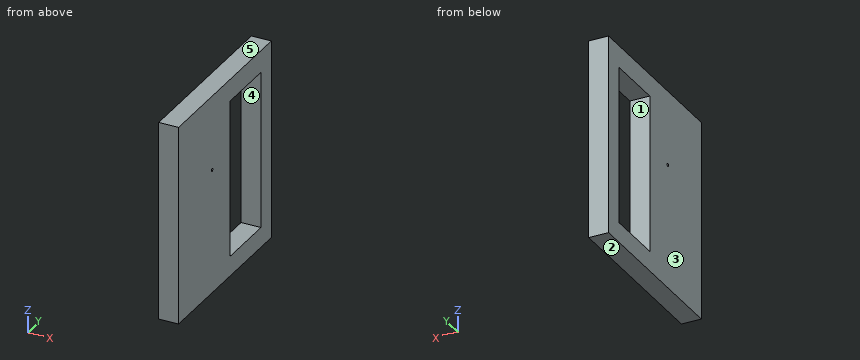
```python
from build123d import *

# Parameters (mm, degrees)
SKETCH4_W           = 25.4
SKETCH4_H           = 228.6
BOSS_EXTRUDE1_DEPTH = 254
CUT_EXTRUDE3_DEPTH  = 280.688487428
SKETCH12_R          = 2
CUT_EXTRUDE4_DEPTH  = 280.688487428


with BuildPart() as part:
    # Sketch4 → Boss-Extrude1 (new body)
    with BuildSketch(Plane.XY):
        Rectangle(SKETCH4_W, SKETCH4_H)
    extrude(amount=BOSS_EXTRUDE1_DEPTH)

    # Sketch11 → Cut-Extrude3 (cut, through all)
    with BuildSketch(Plane(origin=(12.7, 0, 0), x_dir=(0, 0, -1), z_dir=(1, 0, 0))):
        Polygon((-226.0000001, 88.9), (-25.4000001, 88.9), (-25.4, 12.825), (-226.0000001, 12.825), align=None)
    extrude(amount=-CUT_EXTRUDE3_DEPTH, mode=Mode.SUBTRACT)

    # Sketch12 → Cut-Extrude4 (cut, through all)
    with BuildSketch(Plane(origin=(12.7, 0, 0), x_dir=(0, 0, -1), z_dir=(1, 0, 0))):
        with Locations((-158.75, -31.75)):
            Circle(SKETCH12_R)
    extrude(amount=-CUT_EXTRUDE4_DEPTH, mode=Mode.SUBTRACT)


solid = part.part
```
Here's how the part is built. I have some questions about the finished solid (model axes, mm). Face numbers are marked on the shaded views. A direction names the side the tool comes from. Round coordinates to 2 decimals unless told otherwise and drop trailing zeros. Order: outer loops, then holes, each group sorted by start corner. A loop starts at its lowest first (then second) coordinate and runs counter-clockwise, first axis right, second up. Notation, with made-up numbers: (21, 29.25) -> (50, 29.25) arc R16 ccw to (50, 46.25) -> close; hole circle Ø6 at (80, -15.75). An arc over 180 degrees is marked (long way). Use a Markdown table: item, result. Add a question column.
(1) Suppose I cut it at A-A, the plane z = 217.5. Please give me the cut outline in (x, y) (3 decimals), and give its area (3 significant figures).
(2) I need wall thicknesses on line 1 along Z through (x, y) = (-1.5, 72.5); line 2 along Y through (x, z) = (-1.5, 215.5) (3 decimals); line 3 along Y through (x, z) = (2.5, 158.75) (3 decimals). Which ranges of each line are inside material? Lowest first, please.
(3) For the marked faces 4 and 5, which set-ups out of +Z, -Z, +X, -X, +Y, -Y let a thin tool reach every point of the face, with its end or its side?
(4) For pin 1 Ø12 at (x, y) = (-5.5, -43) entering from -Z, with a flat end and sliding along its axis, tell me the tip position at first contact or that it passes through.
(5) If we mould it in two halves opening along Z, with no side actions, what happens to the marked faces 1, 2 and 3? For each: released by +Z, released by -Z, zero draft, split by the parting line, or undercut.
(6) Suppose I cut it at B-B, the plane y = 55. Please give me the cut outline in (x, z).
(7) Suppose I cut it at C-C, the plane x = -1.5. Please give me the cut outline in (y, z) (3 decimals), and give its area (3 significant figures).
Verdict:
| question | item | result |
|---|---|---|
| 1 | outline | (-12.7, -114.3) -> (12.7, -114.3) -> (12.7, 12.825) -> (-12.7, 12.825) -> close; (-12.7, 88.9) -> (12.7, 88.9) -> (12.7, 114.3) -> (-12.7, 114.3) -> close |
| 1 | area | 3,870 mm2 |
| 2 | line 1 | 0 to 25.4, 226 to 254 |
| 2 | line 2 | -114.3 to 12.825, 88.9 to 114.3 |
| 2 | line 3 | -114.3 to -33.75, -29.75 to 12.825, 88.9 to 114.3 |
| 3 | face 4 | +X, -X |
| 3 | face 5 | +Z, +X, -X, +Y, -Y |
| 4 | pin 1 | z = 0 |
| 5 | face 1 | undercut |
| 5 | face 2 | released by -Z |
| 5 | face 3 | zero draft |
| 6 | outline | (-12.7, 0) -> (12.7, 0) -> (12.7, 25.4) -> (-12.7, 25.4) -> close; (-12.7, 226) -> (12.7, 226) -> (12.7, 254) -> (-12.7, 254) -> close |
| 7 | outline | (-114.3, 0) -> (114.3, 0) -> (114.3, 254) -> (-114.3, 254) -> close; hole circle Ø4 at (-31.75, 158.75); hole (12.825, 25.4) -> (88.9, 25.4) -> (88.9, 226) -> (12.825, 226) -> close |
| 7 | area | 42,800 mm2 |
